from build123d import *

# Parameters (mm, degrees)
F0_W     = 5
F0_H     = 8
F0_W_2   = 7
F0_H_2   = 5
F0_W_3   = 1
F0_H_3   = 1
F1_DEPTH = 5
F2_DEPTH = 40
F3_START = 35
F3_DEPTH = 5
F4_DEPTH = 20
F6_D     = 3
F6_DEPTH = 20
F6_TIP   = 0.9012909285


with BuildPart() as f1:
    # F0 (on Top) → F1 (new body)
    with BuildSketch(Plane.XY):
        with Locations((-32.4270167043, 29.4046077263)):
            Rectangle(F0_W, F0_H)
        with Locations((-46.4270167043, 15.9046077263)):
            Rectangle(F0_W_2, F0_H_2)
        with Locations((-52.4270167043, 15.9046077263)):
            Rectangle(F0_W, F0_H_2)
        with Locations((-32.4270167043, 35.9046077263)):
            Rectangle(F0_W, F0_H_2)
        with BuildLine():
            ThreePointArc((-34.9270167043, 15.9046077263), (-34.1947836573, 14.1368407733), (-32.4270167043, 13.4046077263))
            ThreePointArc((-32.4270167043, 13.4046077263), (-30.6592497514, 14.1368407733), (-29.9270167043, 15.9046077263))
            ThreePointArc((-29.9270167043, 15.9046077263), (-30.6592497514, 17.6723746792), (-32.4270167043, 18.4046077263))
            ThreePointArc((-32.4270167043, 18.4046077263), (-34.1947836573, 17.6723746792), (-34.9270167043, 15.9046077263))
        make_face()
        with BuildLine():
            ThreePointArc((-32.4270167043, 18.4046077263), (-30.6592497514, 17.6723746792), (-29.9270167043, 15.9046077263))
            Line((-29.9270167043, 15.9046077263), (-29.9270167043, 18.4046077263))
            Line((-29.9270167043, 18.4046077263), (-32.4270167043, 18.4046077263))
        make_face()
        with BuildLine():
            Line((-34.9270167043, 15.9046077263), (-34.9270167043, 13.4046077263))
            Line((-34.9270167043, 13.4046077263), (-32.4270167043, 13.4046077263))
            ThreePointArc((-32.4270167043, 13.4046077263), (-34.1947836573, 14.1368407733), (-34.9270167043, 15.9046077263))
        make_face()
        with BuildLine():
            ThreePointArc((-29.9270167043, 15.9046077263), (-30.6592497514, 14.1368407733), (-32.4270167043, 13.4046077263))
            Line((-32.4270167043, 13.4046077263), (-29.9270167043, 13.4046077263))
            Line((-29.9270167043, 13.4046077263), (-29.9270167043, 15.9046077263))
        make_face()
        with BuildLine():
            Line((-34.9270167043, 18.4046077263), (-34.9270167043, 15.9046077263))
            ThreePointArc((-34.9270167043, 15.9046077263), (-34.1947836573, 17.6723746792), (-32.4270167043, 18.4046077263))
            Line((-32.4270167043, 18.4046077263), (-34.9270167043, 18.4046077263))
        make_face()
        Polygon((-41.9270167043, 18.4046077263), (-41.9270167043, 13.4046077263), (-34.9270167043, 13.4046077263), (-34.9270167043, 15.9046077263), (-34.9270167043, 18.4046077263), align=None)
        with Locations((-42.4270167043, 15.9046077263)):
            Rectangle(F0_W_3, F0_H_2)
        Polygon((-34.9270167043, 24.4046077263), (-34.9270167043, 18.4046077263), (-32.4270167043, 18.4046077263), (-29.9270167043, 18.4046077263), (-29.9270167043, 24.4046077263), align=None)
        with Locations((-32.4270167043, 24.9046077263)):
            Rectangle(F0_W, F0_H_3)
    extrude(amount=F1_DEPTH)

    # F0 (on Top) → F2 (join)
    with BuildSketch(Plane.XY):
        with Locations((-52.4270167043, 15.9046077263)):
            Rectangle(F0_W, F0_H_2)
        with BuildLine():
            Line((-34.9270167043, 18.4046077263), (-34.9270167043, 15.9046077263))
            ThreePointArc((-34.9270167043, 15.9046077263), (-34.1947836573, 17.6723746792), (-32.4270167043, 18.4046077263))
            Line((-32.4270167043, 18.4046077263), (-34.9270167043, 18.4046077263))
        make_face()
        with BuildLine():
            Line((-34.9270167043, 15.9046077263), (-34.9270167043, 13.4046077263))
            Line((-34.9270167043, 13.4046077263), (-32.4270167043, 13.4046077263))
            ThreePointArc((-32.4270167043, 13.4046077263), (-34.1947836573, 14.1368407733), (-34.9270167043, 15.9046077263))
        make_face()
        with BuildLine():
            ThreePointArc((-34.9270167043, 15.9046077263), (-34.1947836573, 14.1368407733), (-32.4270167043, 13.4046077263))
            ThreePointArc((-32.4270167043, 13.4046077263), (-30.6592497514, 14.1368407733), (-29.9270167043, 15.9046077263))
            ThreePointArc((-29.9270167043, 15.9046077263), (-30.6592497514, 17.6723746792), (-32.4270167043, 18.4046077263))
            ThreePointArc((-32.4270167043, 18.4046077263), (-34.1947836573, 17.6723746792), (-34.9270167043, 15.9046077263))
        make_face()
        with BuildLine():
            ThreePointArc((-32.4270167043, 18.4046077263), (-30.6592497514, 17.6723746792), (-29.9270167043, 15.9046077263))
            Line((-29.9270167043, 15.9046077263), (-29.9270167043, 18.4046077263))
            Line((-29.9270167043, 18.4046077263), (-32.4270167043, 18.4046077263))
        make_face()
        with BuildLine():
            ThreePointArc((-29.9270167043, 15.9046077263), (-30.6592497514, 14.1368407733), (-32.4270167043, 13.4046077263))
            Line((-32.4270167043, 13.4046077263), (-29.9270167043, 13.4046077263))
            Line((-29.9270167043, 13.4046077263), (-29.9270167043, 15.9046077263))
        make_face()
        with Locations((-32.4270167043, 35.9046077263)):
            Rectangle(F0_W, F0_H_2)
        with Locations((-42.4270167043, 15.9046077263)):
            Rectangle(F0_W_3, F0_H_2)
        with Locations((-32.4270167043, 24.9046077263)):
            Rectangle(F0_W, F0_H_3)
    extrude(amount=F2_DEPTH)

    # F0 (on Top) → F3 (join)
    with BuildSketch(Plane.XY.offset(F3_START)):
        with Locations((-32.4270167043, 29.4046077263)):
            Rectangle(F0_W, F0_H)
        with Locations((-46.4270167043, 15.9046077263)):
            Rectangle(F0_W_2, F0_H_2)
        Polygon((-41.9270167043, 18.4046077263), (-41.9270167043, 13.4046077263), (-34.9270167043, 13.4046077263), (-34.9270167043, 15.9046077263), (-34.9270167043, 18.4046077263), align=None)
        Polygon((-34.9270167043, 24.4046077263), (-34.9270167043, 18.4046077263), (-32.4270167043, 18.4046077263), (-29.9270167043, 18.4046077263), (-29.9270167043, 24.4046077263), align=None)
    extrude(amount=F3_DEPTH)

    # F0 (on Top) → F4 (join)
    with BuildSketch(Plane.XY):
        with BuildLine():
            ThreePointArc((-34.9270167043, 15.9046077263), (-34.1947836573, 14.1368407733), (-32.4270167043, 13.4046077263))
            ThreePointArc((-32.4270167043, 13.4046077263), (-30.6592497514, 14.1368407733), (-29.9270167043, 15.9046077263))
            ThreePointArc((-29.9270167043, 15.9046077263), (-30.6592497514, 17.6723746792), (-32.4270167043, 18.4046077263))
            ThreePointArc((-32.4270167043, 18.4046077263), (-34.1947836573, 17.6723746792), (-34.9270167043, 15.9046077263))
        make_face()
    extrude(amount=-F4_DEPTH)

    # F6
    with Locations(Plane.XY.offset(40)):
        with Locations((-44.4270167043, 15.9046077263), (-32.4270167043, 27.9046077263)):
            Hole(F6_D / 2, depth=F6_DEPTH)
            with Locations((0, 0, -(F6_DEPTH + F6_TIP / 2))):  # 118° drill point
                Cone(0, F6_D / 2, F6_TIP, mode=Mode.SUBTRACT)


solid = f1.part
Model file for the job. Use its own axes, mm. A direction names the side the tool comes from. Give positions to 0.01 mm unless a question says otherwise; leave off trailing zeros. Order: outer loops, then holes, each group sorted by start corner. A loop starts at its lowest first (then second) coordinate and runs counter-clockwise, first axis right, second up. Notation, with made-up numbers: (73.25, 83.5) - (89.25, 83.5) arc R14 cw to (89.25, 99.5) - close; hole circle Ø6 at (11.25, 62.25). An arc over 180 degrees is marked (long way). One line per item, written item: value.
Item 1: Tool access for faces 1 (the flat face through (-30.4, 13.9, 0)), 2 (the flat face through (-49.927, 16, 20)), 3 (the cylindrical face through (-30.93, 27.97, 37.47)), 4 (the flat face through (-32, 25.405, 20)): list every direction of +Z, -Z, +X, -X, +Y, -Y with a clear straight run to the whole face (end or side of a thin tool).
Response values:
face 1: -Z, +X, -Y
face 2: +Y, -Y
face 3: +Z
face 4: +X, -X
Item 2: Slice it at C-C (z = 30). List the corners of the cut face in (x, y).
Response values:
outline: (-54.93, 13.4) - (-49.93, 13.4) - (-49.93, 18.4) - (-54.93, 18.4) - close; (-42.93, 13.4) - (-41.93, 13.4) - (-41.93, 18.4) - (-42.93, 18.4) - close; (-34.93, 13.4) - (-29.93, 13.4) - (-29.93, 18.4) - (-34.93, 18.4) - close; (-34.93, 24.4) - (-29.93, 24.4) - (-29.93, 25.4) - (-34.93, 25.4) - close; (-34.93, 33.4) - (-29.93, 33.4) - (-29.93, 38.4) - (-34.93, 38.4) - close
Item 3: Two-plate mould, pull along X, no slides. Class faces 5 (the flat face through (-37, 18, 40)), 6 (the flat face through (-38, 16, 5)), 7 (the flat face through (-54.927, 16, 20)): released by +X, released by -X, zero draft, split by the parting line, or undercut.
Response values:
face 5: zero draft
face 6: undercut
face 7: released by -X
Item 4: Pin check, flat tips, straight feed: pin 1 Ø4 at (x, y) = (-32.5, 28.5) entering from -Z; pin 2 Ø2 at (y, z) = (18.5, -11.5) entering from -X; pin 3 Ø1.5 at (y, z) = (29.5, 3.5) entering from -X. Stop position of each tip, or through.
Response values:
pin 1: z = 0
pin 2: x = -34.35
pin 3: x = -34.93
Item 5: Slice it at A-A (x = -37.25). List the corners of the cut face in (y, z).
Response values:
outline: (13.4, 0) - (18.4, 0) - (18.4, 5) - (13.4, 5) - close; (13.4, 35) - (18.4, 35) - (18.4, 40) - (13.4, 40) - close
Item 6: Slice it at B-B (y = 19.25). List the corners of the cut face in (x, z), then the cut area to 3 significant figures.
Response values:
outline: (-34.93, 0) - (-29.93, 0) - (-29.93, 5) - (-34.93, 5) - close; (-34.93, 35) - (-29.93, 35) - (-29.93, 40) - (-34.93, 40) - close
area: 50.0 mm2
Item 7: Wall check: line 1 (X direction, y = 16.5, z = 24.5); line 2 (Y direction, x = -32.75, z = 23); line 3 (Z direction, x = -34.25, y = 18.5). Give the ranges that are in metal, low to high.
Response values:
line 1: -54.93 to -49.93, -42.93 to -41.93, -34.93 to -29.93
line 2: 13.4 to 18.4, 24.4 to 25.4, 33.4 to 38.4
line 3: 0 to 5, 35 to 40
Item 8: Slice it at D-D (y = 16.75). List the corners of the cut face in (x, z), then the cut area to 3 significant figures.
Response values:
outline: (-54.93, 0) - (-34.78, 0) - (-34.78, -20) - (-30.07, -20) - (-30.07, 0) - (-29.93, 0) - (-29.93, 40) - (-43.19, 40) - (-43.19, 35) - (-42.93, 35) - (-42.93, 5) - (-49.93, 5) - (-49.93, 35) - (-45.67, 35) - (-45.67, 40) - (-54.93, 40) - close; hole (-41.93, 5) - (-34.93, 5) - (-34.93, 35) - (-41.93, 35) - close
area: 662 mm2
